Autodesk Inventor part; units mm, degrees
ref_plane "YZ Plane" through (0, 0, 0) normal (1, 0, 0) x (0, 1, 0)
ref_plane "XZ Plane" through (0, 0, 0) normal (0, 1, 0) x (-1, 0, 0)
ref_plane "XY Plane" through (0, 0, 0) normal (0, 0, 1) x (1, 0, 0)
sketch "Boceto1" plane through (0, 0, 0) normal (0, 1, 0) x (-1, 0, 0)
  circle A0 centre (0, 0) radius 5
  dimension "d0" = 10
extrude "Extrusión1" add sketch "Boceto1" along normal blind 3
sketch "Boceto2" plane through (0, 3, 0) normal (0, 1, 0) x (1, 0, 0)
  circle A0 centre (0, 0) radius 2.5
  dimension "d3" = 5
extrude "Extrusión2" cut sketch "Boceto2" against normal through all
fillet "Empalme1" radius 1.5 2 edges at (5, 3, 0) (5, 0, 0)
properties part number "shocks_rubber" material "Goma"
Check sheet for the modelled part. Datum: model origin and axes. Units: mm. Coordinates: 2 decimals unless noted, no trailing zeros. Order: outer loops, then holes, each group sorted by start corner. A loop starts at its lowest first (then second) coordinate and runs counter-clockwise, first axis right, second up. Notation, with made-up numbers: (-33, -18.5) -> (-5, -18.5) arc R19 cw to (-5, 9.5) -> close; hole circle Ø5 at (-32.5, 86). An arc over 180 degrees is marked (long way). Write each question's results on one line, items separated by ' | '. Start each with the question number.
1) Draft check along Z on faces 1 (the face through (-0.54, 1.52, 2.44)), 2 (the face through (-2, 3, -2)). Enter one of: pulls with the +Z half, pulls with the -Z half, needs draft (parallel to the pull), parting line crosses it, or undercut.
2) Section check B-B (y = 0.7). Enter the section's corners in (x, z).
3) Section check C-C (y = 1.25). Enter the section's corners in (x, z), and give its area (3 significant figures).
4) Material ranges on line 1 along Z through (x, y) = (0, 1.85); line 2 along X through (y, z) = (0.75, -0.75); line 3 along Z through (x, y) = (1.5, 1.7), recorded low to high.
Checked values:
1) face 1: undercut | face 2: needs draft
2) outline: circle Ø9.54 at (0, 0); hole circle Ø5 at (0, 0)
3) outline: circle Ø9.96 at (0, 0); hole circle Ø5 at (0, 0) | area: 58.2 mm²
4) line 1: -4.96 to -2.5, 2.5 to 4.96 | line 2: -4.74 to -2.38, 2.38 to 4.74 | line 3: -4.76 to -2, 2 to 4.76
